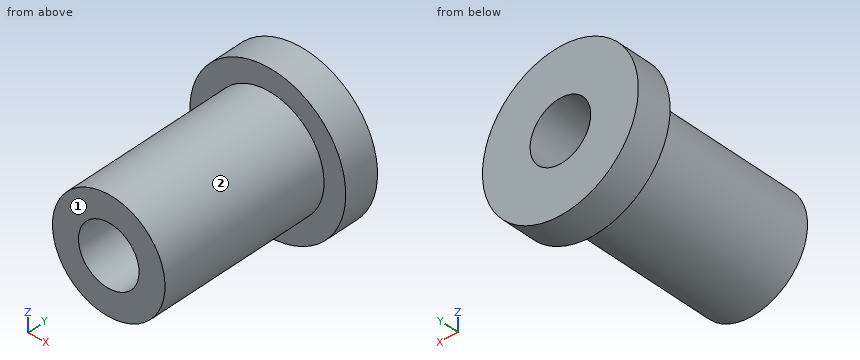
```python
from build123d import *

# Parameters (mm, degrees)
SKETCH1_R           = 4.5
BOSS_EXTRUDE1_DEPTH = 12
SKETCH3_R           = 4.5
SKETCH3_R_2         = 3.25
CUT_EXTRUDE1_DEPTH  = 10
SKETCH4_R           = 1.75
CUT_EXTRUDE2_DEPTH  = 12


with BuildPart() as part:
    # Sketch1 → Boss-Extrude1 (new body)
    with BuildSketch(Plane(origin=(0, 0, 0), x_dir=(1, 0, 0), z_dir=(0, 1, 0))):
        with Locations(Location((0, 0, 0), (0, 0, 270))):
            Circle(SKETCH1_R)
    extrude(amount=BOSS_EXTRUDE1_DEPTH)

    # Sketch3 → Cut-Extrude1 (cut)
    with BuildSketch(Plane(origin=(0, 0, 0), x_dir=(-1, 0, 0), z_dir=(0, -1, 0))):
        with Locations(Location((0, 0, 0), (0, 0, 90))):
            Circle(SKETCH3_R)
        with Locations(Location((0, 0, 0), (0, 0, 90))):
            Circle(SKETCH3_R_2, mode=Mode.SUBTRACT)
    extrude(amount=-CUT_EXTRUDE1_DEPTH, mode=Mode.SUBTRACT)

    # Sketch4 → Cut-Extrude2 (cut)
    with BuildSketch(Plane(origin=(0, 0, 0), x_dir=(-1, 0, 0), z_dir=(0, -1, 0))):
        with Locations(Location((0, 0, 0), (0, 0, 90))):
            Circle(SKETCH4_R)
    extrude(amount=-CUT_EXTRUDE2_DEPTH, mode=Mode.SUBTRACT)


solid = part.part
```
Can you work these out from the model? Positions are in its coordinate system, mm. Face numbers are marked on the shaded views. A direction names the side the tool comes from. Coordinates: 2 decimals unless noted, no trailing zeros. Loops run counter-clockwise (first coordinate to the right, second up) from the corner with the lowest first, then second, coordinate; pieces in that order, holes last.
1) Imagine slicing it at D-D on y = 6.25. List the corners of the cut face in (x, z) for me, plus the area to 3 significant figures.
2) Which directions (+Z, -Z, +X, -X, +Y, -Y) give clear straight access to the entire face, cutting with the end or side of a thin tool? Please do the marked faces 1 and 2.
3) Imagine slicing it at A-A on z = 0. List the corners of the cut face in (x, y) for me.
4) Imagine slicing it at B-B on x = 0. List the corners of the cut face in (y, z) for me, plus the area to 3 significant figures.
5) For pin 1 (1.5 mm diameter, centred on y = 3, z = -1.5, fed in from +X); pin 2 (2 mm diameter, centred on x = 0.5, y = 2.5, fed in from -Z); pin 3 (1.5 mm diameter, centred on x = 2, z = -2.5, fed in from -Y); pin 4 (1.5 mm diameter, centred on x = -1.5, y = 8.5, fed in from +Z), each with a flat end and sliding along its axis, tell me the tip position at first contact or that it passes through.
6) Imagine slicing it at C-C on z = 2.25. List the corners of the cut face in (x, y) for me, plus the area to 3 significant figures.
7) I need wall thicknesses on probe 1 along X at (y, z) = (9.5, 0); probe 2 along Y at (x, z) = (2.75, 3); probe 3 along Z at (x, y) = (0.25, 7). Which ranges of each line are inside material? Lowest first, please.
Completed:
1. outline: circle Ø6.5 at (0, 0); hole circle Ø3.5 at (0, 0)
1. area: 23.6 mm2
2. face 1: +Z, -Z, +X, -X, -Y
2. face 2: -Y
3. outline: (-4.5, 10) - (-3.25, 10) - (-3.25, 0) - (-1.75, 0) - (-1.75, 12) - (-4.5, 12) - close; (1.75, 0) - (3.25, 0) - (3.25, 10) - (4.5, 10) - (4.5, 12) - (1.75, 12) - close
4. outline: (0, -3.25) - (10, -3.25) - (10, -4.5) - (12, -4.5) - (12, -1.75) - (0, -1.75) - close; (0, 1.75) - (12, 1.75) - (12, 4.5) - (10, 4.5) - (10, 3.25) - (0, 3.25) - close
4. area: 41.0 mm2
5. pin 1: stops at x = 3.16
5. pin 2: stops at z = -3.25
5. pin 3: stops at y = 0
5. pin 4: stops at z = 3.16
6. outline: (-3.9, 10) - (-2.35, 10) - (-2.35, 0) - (2.35, 0) - (2.35, 10) - (3.9, 10) - (3.9, 12) - (-3.9, 12) - close
6. area: 62.5 mm2
7. probe 1: x = -3.25 to -1.75, 1.75 to 3.25
7. probe 2: y = 10 to 12
7. probe 3: z = -3.24 to -1.73, 1.73 to 3.24
